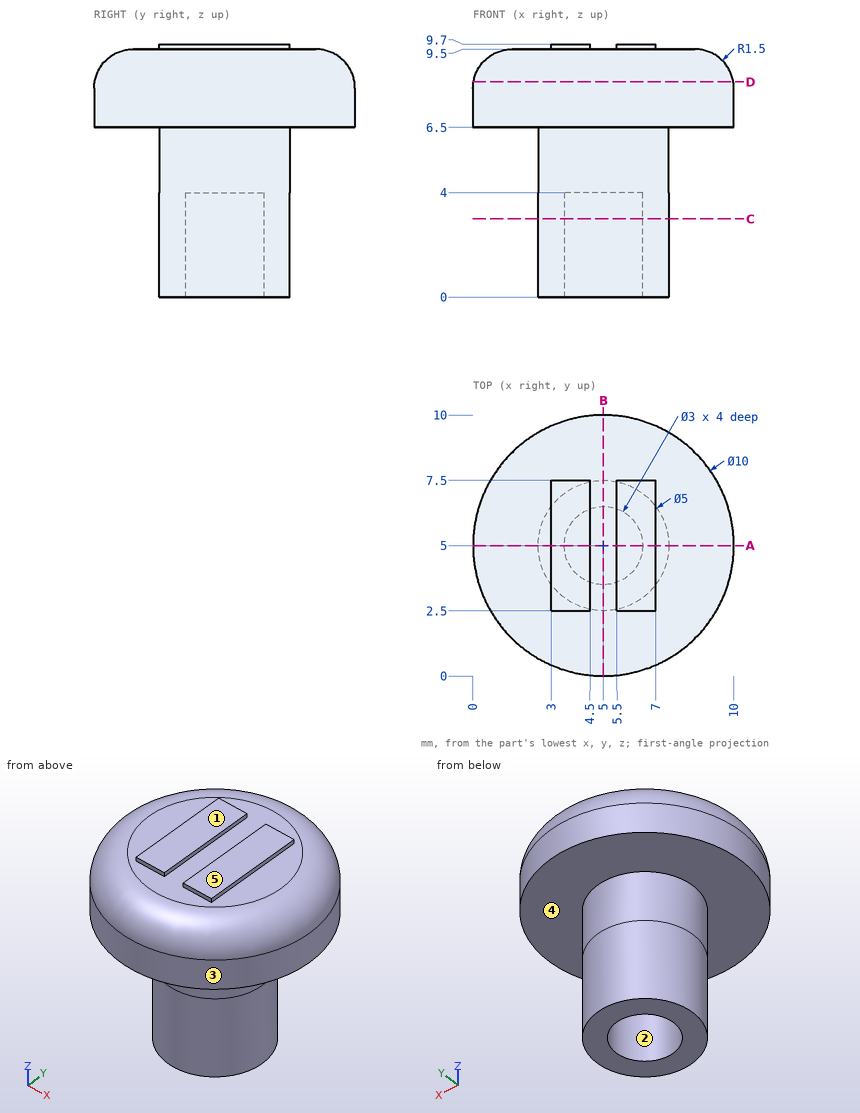
Print and shaded views of the part. All mm, measured from the part's lowest x, y and z. A direction names the side the tool comes from. Coordinates: 2 decimals unless noted, no trailing zeros. Order: outer loops, then holes, each group sorted by start corner. A loop starts at its lowest first (then second) coordinate and runs counter-clockwise, first axis right, second up. Notation, with made-up numbers: M -19,68.5 L 4,68.5 A17 cw 4,74.5 Z; hole C 76,4 d2. An arc over 180 degrees is marked long. One line per question, with ' | ' between items. Start each with the question number.
Q1. Saw through at C-C (z = 3). List the corners of the cut face in (x, y), then the cut area to 3 significant figures.
Q2. Two-plate mould, pull along X, no slides. Class the marked faces 1, 2 and 3: +X half, -X half, draft (parallel to the pull), parting line (faces both ways), or undercut.
Q3. Saw through at D-D (z = 8.25). List the corners of the cut face in (x, y).
Q4. Probe L1, parallel to X at y = 5, z = 2.8; L2, parallel to Z at x = 2.25, y = 2.75. List the from-to ranges inside material, lowest first. Write a range as from..to.
Q5. Saw through at A-A (y = 5). List the corners of the cut face in (x, z).
Q6. Saw through at B-B (x = 5). List the corners of the cut face in (y, z).
Q7. 3-axis set-ups, long thin cutter, end or side, ignore diameter. For the marked faces 4 and 5: which of +Z, -Z, +X, -X, +Y, -Y reach the whole face in a straight line?
Q8. Flat gauge pin, fed straight in: pin 1 Ø0.9 at (x, y) = (5, 5) entering from -Z. Where does the tip first touch, or does it go through?
Check values:
1) outline: C 5,5 d5; hole C 5,5 d3 | area: 12.6 mm2
2) face 1: draft | face 2: undercut | face 3: parting line
3) outline: C 5,5 d9.96
4) L1: x = 2.5..3.5, 6.5..7.5 | L2: z = 6.5..9.5
5) outline: M 0,6.5 L 2.5,6.5 L 2.5,0 L 3.5,0 L 3.5,4 L 6.5,4 L 6.5,0 L 7.5,0 L 7.5,6.5 L 10,6.5 L 10,8 A1.5 ccw 8.5,9.5 L 7,9.5 L 7,9.7 L 5.5,9.7 L 5.5,9.5 L 4.5,9.5 L 4.5,9.7 L 3,9.7 L 3,9.5 L 1.5,9.5 A1.5 ccw 0,8 Z
6) outline: M 0,6.5 L 2.5,6.5 L 2.5,0 L 3.5,0 L 3.5,4 L 6.5,4 L 6.5,0 L 7.5,0 L 7.5,6.5 L 10,6.5 L 10,8 A1.5 ccw 8.5,9.5 L 1.5,9.5 A1.5 ccw 0,8 Z
7) face 4: -Z | face 5: +Z, +X, -X, +Y, -Y
8) pin 1: stops at z = 4
